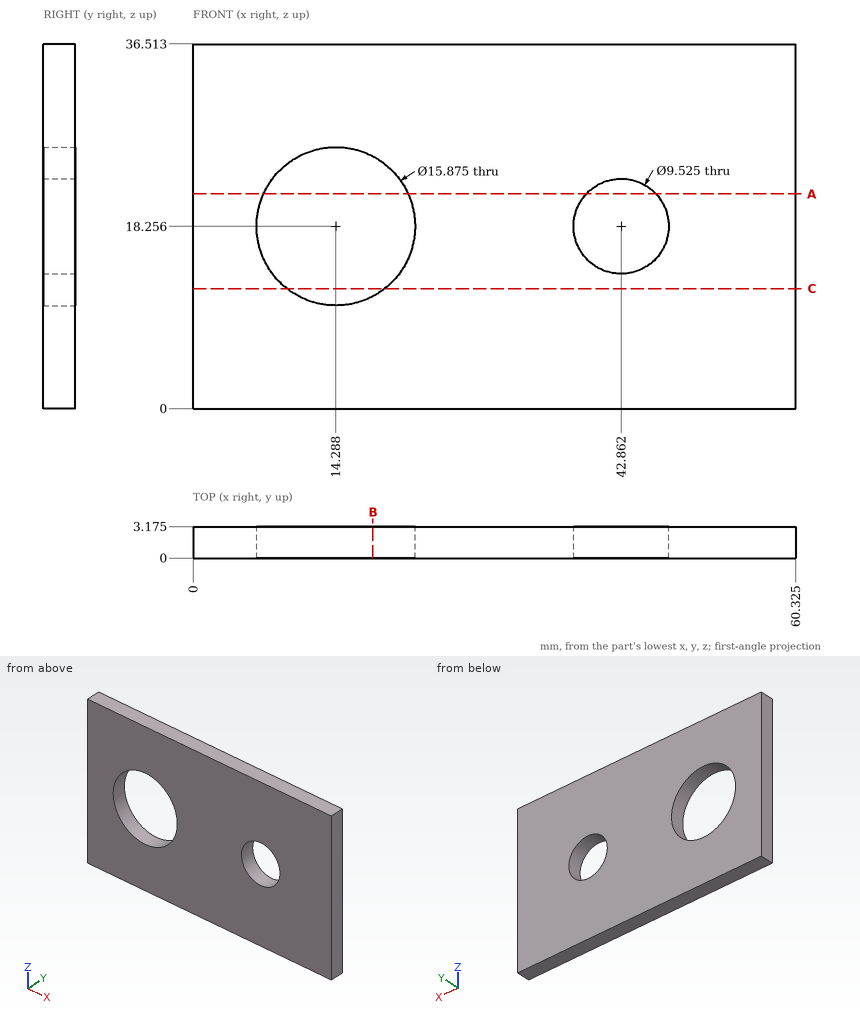
The figure shows three views and two pictorial views of one solid part (mm, origin at its lowest corner). Answer the questions. Round coordinates to 2 decimals unless told otherwise and drop trailing zeros. Loops run counter-clockwise (first coordinate to the right, second up) from the corner with the lowest first, then second, coordinate; pieces in that order, holes last. Notation, with made-up numbers: M 22,9 L 61,9 A15 ccw 61,21 Z; hole C 45.25,51 d9. An arc over 180 degrees is marked long. Write each question's results on one line, items separated by ' | '. Start each with the question number.
1) Straight lines are drawn through the part: probe 1 along X at (y, z) = (0.85, 20) (1 decimal); probe 2 along Z at (x, y) = (43, 2.1) (1 decimal); probe 3 along X at (y, z) = (1.75, 22) (1 decimal). For each, find the intervals that lie inside material, in ascending order.
2) Find section C-C on z = 12. Write down the section's boundary in (x, y) (1 decimal).
3) This flat-tipped pin is pushed along its axis until it touches: pin 1 (9.5 mm diameter, centred on x = 14.29, z = 18.26, fed in from +Y). Where does it stop, or does it pass through?
4) Find section B-B on x = 18. Write down the section's boundary in (y, z) (1 decimal).
5) Find section A-A on z = 21.5. Count the separate pieces of the cut face and the enclosed holes in it, plus the area to 3 significant figures.
Final values:
1) probe 1: 0 to 6.5, 22 to 38.4, 47.3 to 60.3 | probe 2: 0 to 13.5, 23 to 36.5 | probe 3: 0 to 7.3, 21.3 to 39.9, 45.8 to 60.3
2) outline: M 0,0 L 9.4,0 L 9.4,3.2 L 0,3.2 Z; M 19.2,0 L 60.3,0 L 60.3,3.2 L 19.2,3.2 Z
3) pin 1: through
4) outline: M 0,0 L 3.2,0 L 3.2,11.2 L 0,11.2 Z; M 0,25.3 L 3.2,25.3 L 3.2,36.5 L 0,36.5 Z
5) separate pieces: 3 | enclosed holes: 0 | area: 123 mm²
